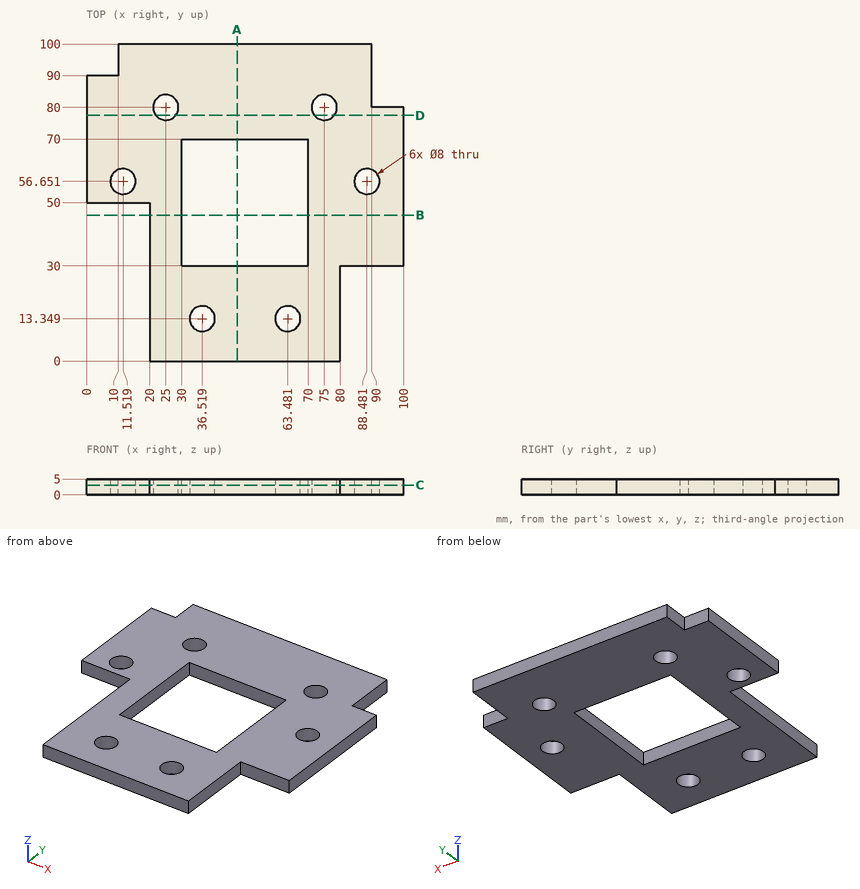
Check sheet for the drawn part. Datum: minimum x, y, z corner. Units: mm. Round coordinates to 2 decimals unless told otherwise and drop trailing zeros. Loops run counter-clockwise (first coordinate to the right, second up) from the corner with the lowest first, then second, coordinate; pieces in that order, holes last. Notation, with made-up numbers: (39.25, 51.25) -> (62.25, 51.25) arc R36 cw to (62.25, 87.25) -> close; hole circle Ø3 at (-17.75, 30.25). An arc over 180 degrees is marked (long way). Put each result on its own line as item: value. Start each with the question number.
1. Section check A-A (x = 47.5). Enter the section's corners in (y, z).
2. Section check D-D (y = 77.5). Enter the section's corners in (x, z).
3. Section check C-C (z = 3.05). Enter the section's corners in (x, y), plus the area to 3 significant figures.
4. Section check B-B (y = 46). Enter the section's corners in (x, z), plus the area to 3 significant figures.
5. Gauge pin test, flat ends, axial feed: pin 1 (2.5 mm diameter, centred on y = 93, z = 2, fed in from -X); pin 2 (2.5 mm diameter, centred on x = 87, z = 1.5, fed in from -Y); pin 3 (1.5 mm diameter, centred on y = 27, z = 2.5, fed in from -X). Record the tip position at first contact, or that the pin passes through.
6. Scan lines: probe 1 along X at (y, z) = (40.5, 2.95); probe 2 along Y at (x, z) = (75, 1.6); probe 3 along Y at (x, z) = (56.5, 1.5). Record each from-to range of solid material in increasing order.
Findings:
1. outline: (0, 0) -> (30, 0) -> (30, 5) -> (0, 5) -> close; (70, 0) -> (100, 0) -> (100, 5) -> (70, 5) -> close
2. outline: (0, 0) -> (21.88, 0) -> (21.88, 5) -> (0, 5) -> close; (28.12, 0) -> (71.88, 0) -> (71.88, 5) -> (28.12, 5) -> close; (78.12, 0) -> (100, 0) -> (100, 5) -> (78.12, 5) -> close
3. outline: (0, 50) -> (20, 50) -> (20, 0) -> (80, 0) -> (80, 30) -> (100, 30) -> (100, 80) -> (90, 80) -> (90, 100) -> (10, 100) -> (10, 90) -> (0, 90) -> close; hole circle Ø8 at (11.52, 56.65); hole circle Ø8 at (25, 80); hole (30, 30) -> (70, 30) -> (70, 70) -> (30, 70) -> close; hole circle Ø8 at (36.52, 13.35); hole circle Ø8 at (63.48, 13.35); hole circle Ø8 at (75, 80); hole circle Ø8 at (88.48, 56.65)
3. area: 6,200 mm^2
4. outline: (20, 0) -> (30, 0) -> (30, 5) -> (20, 5) -> close; (70, 0) -> (100, 0) -> (100, 5) -> (70, 5) -> close
4. area: 200 mm^2
5. pin 1: stops at x = 10
5. pin 2: stops at y = 30
5. pin 3: stops at x = 20
6. probe 1: x = 20 to 30, 70 to 100
6. probe 2: y = 0 to 76, 84 to 100
6. probe 3: y = 0 to 30, 70 to 100
